The figure shows three views and two pictorial views of one solid part (mm, origin at its lowest corner). Answer the questions. Coordinates: 2 decimals unless noted, no trailing zeros. Loops run counter-clockwise (first coordinate to the right, second up) from the corner with the lowest first, then second, coordinate; pieces in that order, holes last. Notation, with made-up numbers: (22.25, 85.25) - (49.25, 85.25) arc R18 ccw to (49.25, 96.25) - close; hole circle Ø3 at (28.25, -13.75). An arc over 180 degrees is marked (long way). One line per question, with ' | ' between items.
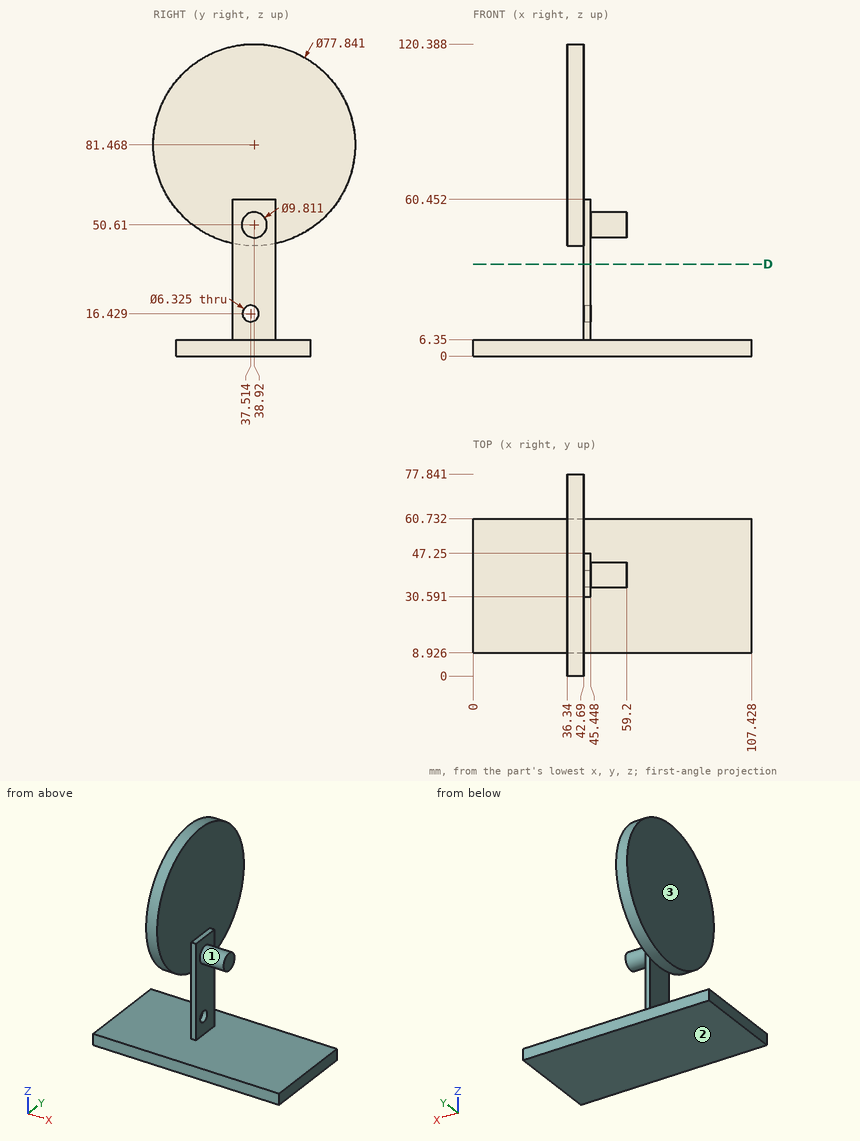
Item 1: Find the intervals of material crossed by line 1 (X direction, y = 43.5, z = 20); line 2 (Z direction, x = 65, y = 58); line 3 (X direction, y = 43, z = 103), in increasing order. Write a range as [from, to].
Taken from the geometry:
line 1: x = [42.69, 45.45] | line 2: z = [0, 6.35] | line 3: x = [36.34, 42.69]
Item 2: Find section D-D, the plane z = 35.5. Write down the section's boundary in (x, y).
Taken from the geometry:
outline: (42.69, 30.59) - (45.45, 30.59) - (45.45, 47.25) - (42.69, 47.25) - close
Item 3: The mould has two halves that part along Z. Classify the marked faces 1, 2 and 3: pulls with the +Z half, pulls with the -Z half, needs draft (parallel to the pull), parting line crosses it, or undercut.
Taken from the geometry:
face 1: undercut | face 2: pulls with the -Z half | face 3: needs draft
Item 4: Each of these flat-tipped pins is pushed along its axis until it touches: pin 1 Ø10 at (x, y) = (86, 21.5) entering from -Z; pin 2 Ø0.8 at (x, z) = (44, 23) entering from +Y; pin 3 Ø7 at (x, z) = (79.5, 1.5) entering from +Y; pin 4 Ø1.5 at (y, z) = (63.5, 55.5) entering from +X. Where does it stop, or does it pass through?
Taken from the geometry:
pin 1: stops at z = 0 | pin 2: stops at y = 47.25 | pin 3: stops at y = 60.73 | pin 4: stops at x = 42.69
